Could you check a few things on this model? Use its own coordinates, in mm. A direction names the side the tool comes from. Give positions to 0.01 mm unless a question says otherwise; leave off trailing zeros. Loops run counter-clockwise (first coordinate to the right, second up) from the corner with the lowest first, then second, coordinate; pieces in that order, holes last. Notation, with made-up numbers: (-32.5, 61) -> (14.5, 61) arc R19 ccw to (14.5, 87) -> close; hole circle Ø3 at (56, 80.25). An arc over 180 degrees is marked (long way). Write item = value, one per line. Start each with the question number.
1) On a 3-axis mill with a long thin cutter (end or side, diameter ignored), from which of +Z, -Z, +X, -X, +Y, -Y can I reach the whole of each face in a straight line? I mean faces 1 (the face through (-11, 46.609, -26)), 2 (the face through (4, 51.689, -19)), 3 (the face through (0, 19, -29.4)), 4 (the face through (0, 42.799, -33)), 5 (the face through (0, 48, 17.97)). Say none if no direction works.
2) I want a section at C-C (y = 12). List the corners of the cut face in (x, z) for me, and give its area (3 significant figures).
3) I want a section at D-D (x = -4.25). List the corners of the cut face in (y, z) for me.
4) I need wall thicknesses on probe 1 along Z at (x, y) = (1.75, 19.5); probe 2 along Y at (x, z) = (-10.25, -3); probe 3 along Y at (x, z) = (6.5, 30). Which ranges of each line are inside material? Lowest first, please. Write a range as from..to.
5) I'm going to push flat-ended pins straight in: pin 1 Ø3.5 at (x, y) = (6.5, 47.5) entering from +Z; pin 2 Ø9 at (x, z) = (-3.5, 23) entering from +Y; pin 3 Ø2.5 at (x, z) = (3, 34) entering from +Y. Where does each tip first touch, or does it pass through?
6) I want a section at B-B (z = 5.5). List the corners of the cut face in (x, y) for me, and give its area (3 significant figures).
7) I want a section at A-A (x = 11.5). List the corners of the cut face in (y, z) for me.
from build123d import *

# Parameters (mm, degrees)
SKETCH2_W           = 28.575
SKETCH2_H           = 58.801
BOSS_EXTRUDE1_DEPTH = 46.609
BOSS_EXTRUDE2_START = -3.81
SKETCH3_W           = 28.575
SKETCH3_H           = 74.041
BOSS_EXTRUDE2_DEPTH = 3.81
BOSS_EXTRUDE3_DEPTH = 3.175
SKETCH5_R           = 6.9215
BOSS_EXTRUDE4_DEPTH = 1.905
SKETCH6_R           = 5.3975
BOSS_EXTRUDE5_DEPTH = 7.62


with BuildPart() as part:
    # Sketch2 → Boss-Extrude1 (new body)
    with BuildSketch(Plane(origin=(0, 0, 0), x_dir=(1, 0, 0), z_dir=(0, 1, 0))):
        Rectangle(SKETCH2_W, SKETCH2_H)
    extrude(amount=BOSS_EXTRUDE1_DEPTH)

    # Sketch3 → Boss-Extrude2 (add)
    with BuildSketch(Plane(origin=(0, 46.609, 0), x_dir=(1, 0, 0), z_dir=(0, 1, 0)).offset(BOSS_EXTRUDE2_START)):
        Rectangle(SKETCH3_W, SKETCH3_H)
    extrude(amount=-BOSS_EXTRUDE2_DEPTH)

    # Sketch4 → Boss-Extrude3 (add)
    with BuildSketch(Plane(origin=(0, 46.609, 0), x_dir=(1, 0, 0), z_dir=(0, 1, 0))):
        with BuildLine():
            Line((-14.2875, 15.113), (-14.2875, -17.9705))
            Line((-14.2875, -17.9705), (14.2875, -17.9705))
            Line((14.2875, -17.9705), (14.2875, 15.113))
            ThreePointArc((14.2875, 15.113), (0, 29.4005), (-14.2875, 15.113))
        make_face()
    extrude(amount=BOSS_EXTRUDE3_DEPTH)

    # Sketch5 → Boss-Extrude4 (add)
    with BuildSketch(Plane(origin=(0, 49.784, 0), x_dir=(1, 0, 0), z_dir=(0, 1, 0))):
        with Locations(Location((0, 15.0495, 0), (0, 0, 90))):
            Circle(SKETCH5_R)
    extrude(amount=BOSS_EXTRUDE4_DEPTH)

    # Sketch6 → Boss-Extrude5 (add)
    with BuildSketch(Plane(origin=(0, 51.689, 0), x_dir=(1, 0, 0), z_dir=(0, 1, 0))):
        with Locations(Location((0, 15.0495, 0), (0, 0, 90))):
            Circle(SKETCH6_R)
    extrude(amount=BOSS_EXTRUDE5_DEPTH)


solid = part.part
Answer list:
q1.face_1 = -Z, -X, +Y
q1.face_2 = +Y
q1.face_3 = -Z, +X, -X, -Y
q1.face_4 = -Z, +X, -X, +Y
q1.face_5 = +Z, +X, -X, +Y
q2.outline = (-14.29, -29.4) -> (14.29, -29.4) -> (14.29, 29.4) -> (-14.29, 29.4) -> close
q2.area = 1,680 mm^2
q3.outline = (0, -29.4) -> (38.99, -29.4) -> (38.99, -37.02) -> (42.8, -37.02) -> (42.8, -29.4) -> (46.61, -29.4) -> (46.61, -28.75) -> (49.78, -28.75) -> (49.78, -20.51) -> (51.69, -20.51) -> (51.69, -18.38) -> (59.31, -18.38) -> (59.31, -11.72) -> (51.69, -11.72) -> (51.69, -9.59) -> (49.78, -9.59) -> (49.78, 17.97) -> (46.61, 17.97) -> (46.61, 29.4) -> (42.8, 29.4) -> (42.8, 37.02) -> (38.99, 37.02) -> (38.99, 29.4) -> (0, 29.4) -> close
q4.probe_1 = -29.4..29.4
q4.probe_2 = 0..49.78
q4.probe_3 = 38.99..42.8
q5.pin_1 = 29.4
q5.pin_2 = 46.61
q5.pin_3 = 42.8
q6.outline = (-14.29, 0) -> (14.29, 0) -> (14.29, 49.78) -> (-14.29, 49.78) -> close
q6.area = 1,420 mm^2
q7.outline = (0, -29.4) -> (38.99, -29.4) -> (38.99, -37.02) -> (42.8, -37.02) -> (42.8, -29.4) -> (46.61, -29.4) -> (46.61, -23.59) -> (49.78, -23.59) -> (49.78, 17.97) -> (46.61, 17.97) -> (46.61, 29.4) -> (42.8, 29.4) -> (42.8, 37.02) -> (38.99, 37.02) -> (38.99, 29.4) -> (0, 29.4) -> close
